Geometry: final body of the model. Coordinates: model frame, mm. Give positions to 0.01 mm unless a question says otherwise; leave off trailing zeros. Write each loop counter-clockwise with the first axis right and the second up, starting at its lowest first coordinate (ties: lowest second). Pieces come first, ordered by that corner, then holes. Notation, with made-up numbers: (8.5, 53.5) -> (55.5, 53.5) arc R18 cw to (55.5, 77.5) -> close; hole circle Ø6 at (28, -0.5). An arc over 180 degrees is marked (long way). Answer as a JSON object with one key per item and string values.
from build123d import *

# Parameters (mm, degrees)
F0_W     = 200
F0_H     = 200
F1_DEPTH = 5
F2_W     = 15.64841
F2_H     = 4
F2_W_2   = 4
F2_H_2   = 15.764192
F3_DEPTH = 25


with BuildPart() as f1:
    # F0 (on Front) → F1 (new body)
    with BuildSketch(Plane.XZ):
        Rectangle(F0_W, F0_H)
    extrude(amount=F1_DEPTH)

    # F2 (on face) → F3 (cut)
    with BuildSketch(Plane.XZ.offset(5)):
        with Locations((-83.275795, 93.1)):
            Rectangle(F2_W, F2_H)
        with Locations((-50.275795, 93.1)):
            Rectangle(F2_W, F2_H)
        with Locations((-17.275795, 93.1)):
            Rectangle(F2_W, F2_H)
        with Locations((15.724205, 93.1)):
            Rectangle(F2_W, F2_H)
        with Locations((48.724205, 93.1)):
            Rectangle(F2_W, F2_H)
        with Locations((81.724205, 93.1)):
            Rectangle(F2_W, F2_H)
        with Locations((-83.275795, -93.1)):
            Rectangle(F2_W, F2_H)
        with Locations((-50.275795, -93.1)):
            Rectangle(F2_W, F2_H)
        with Locations((-17.275795, -93.1)):
            Rectangle(F2_W, F2_H)
        with Locations((15.724205, -93.1)):
            Rectangle(F2_W, F2_H)
        with Locations((48.724205, -93.1)):
            Rectangle(F2_W, F2_H)
        with Locations((81.724205, -93.1)):
            Rectangle(F2_W, F2_H)
        with Locations((93.1, 81.039183)):
            Rectangle(F2_W_2, F2_H_2)
        with Locations((93.173537, 48.639266)):
            Rectangle(F2_W_2, F2_H_2)
        with Locations((93.247075, 16.23935)):
            Rectangle(F2_W_2, F2_H_2)
        with Locations((93.320613, -16.160567)):
            Rectangle(F2_W_2, F2_H_2)
        with Locations((93.39415, -48.560483)):
            Rectangle(F2_W_2, F2_H_2)
        with Locations((93.467688, -80.9604)):
            Rectangle(F2_W_2, F2_H_2)
        with Locations((-93.1, 81.039183)):
            Rectangle(F2_W_2, F2_H_2)
        with Locations((-93.173537, 48.639266)):
            Rectangle(F2_W_2, F2_H_2)
        with Locations((-93.247075, 16.23935)):
            Rectangle(F2_W_2, F2_H_2)
        with Locations((-93.320613, -16.160567)):
            Rectangle(F2_W_2, F2_H_2)
        with Locations((-93.39415, -48.560483)):
            Rectangle(F2_W_2, F2_H_2)
        with Locations((-93.467688, -80.9604)):
            Rectangle(F2_W_2, F2_H_2)
    extrude(amount=-F3_DEPTH, mode=Mode.SUBTRACT)


solid = f1.part
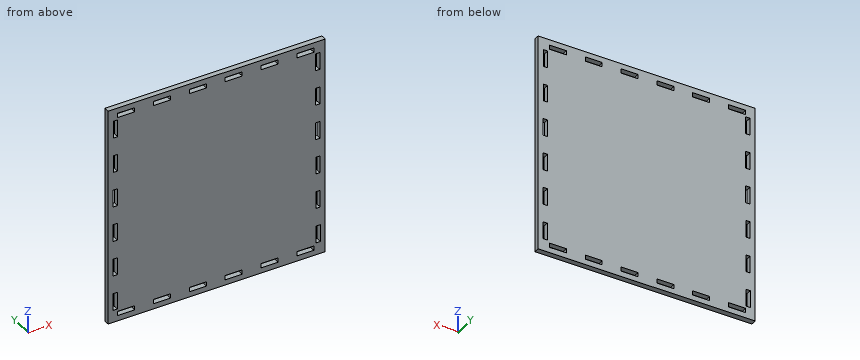
Q1. Cut plane B-B (z = -47). Return the cut outline in (x, y), and give its area (3 significant figures).
Values:
{"outline": "(-100, -5) -> (-95.39, -5) -> (-95.39, 0) -> (-100, 0) -> close; (-91.39, -5) -> (91.39, -5) -> (91.39, 0) -> (-91.39, 0) -> close; (95.39, -5) -> (100, -5) -> (100, 0) -> (95.39, 0) -> close", "area": "960 mm²"}
Q2. Cut plane A-A (x = 84). Return the cut outline in (y, z), and give its area (3 significant figures).
Values:
{"outline": "(-5, -100) -> (0, -100) -> (0, -95.1) -> (-5, -95.1) -> close; (-5, -91.1) -> (0, -91.1) -> (0, 91.1) -> (-5, 91.1) -> close; (-5, 95.1) -> (0, 95.1) -> (0, 100) -> (-5, 100) -> close", "area": "960 mm²"}
Q3. Material intervals for L1, parallel to X at y = -0.55, z = 14; L2, parallel to Z at x = 74, y = -3; L3, parallel to X at y = -2.2, z = -81.5, sorted ascending. Write a range as from..to.
Values:
{"L1": "-100..-95.25, -91.25..91.25, 95.25..100", "L2": "-100..-95.1, -91.1..91.1, 95.1..100", "L3": "-100..-95.47, -91.47..91.47, 95.47..100"}
Q4. Cut plane C-C (y = -2.95). State how many separate pieces and enclosed holes the cut face has, and give its area (3 significant figures).
Values:
{"separate pieces": "1", "enclosed holes": "24", "area": "38,500 mm²"}
